Could you check a few things on this drawing? It's one solid part, dimensions in mm from its lowest x, y, z. A direction names the side the tool comes from. Give positions to 0.01 mm unless a question says otherwise; leave off trailing zeros. Order: outer loops, then holes, each group sorted by start corner. A loop starts at its lowest first (then second) coordinate and runs counter-clockwise, first axis right, second up.
Item 1: I want a section at D-D, the plane z = 12.5. Write out the boundary of the cut face in (x, y).
Item 2: I'm going to push flat-ended pins straight in: pin 1 Ø3.5 at (x, z) = (22, 7.5) entering from +Y; pin 2 Ø5 at (x, y) = (14.5, 12) entering from -Z. Where does each tip first touch, or does it pass through?
Item 3: I want a section at A-A, the plane y = 7.5. Write out the boundary of the cut face in (x, z), then the cut area to 3 significant figures.
Item 4: I want a section at B-B, the plane z = 2.4. Write out the boundary of the cut face in (x, y).
Item 5: Which directions (+Z, -Z, +X, -X, +Y, -Y) give clear straight access to the entire face, cutting with the end or side of a thin tool? Please do the marked faces 5, 6 and 7.
Item 6: I want a section at C-C, the plane x = 21. Write out the boundary of the cut face in (y, z), then the cut area to 3 significant figures.
Item 7: If I drill on line 1 along Z through (x, y) = (2.4, 1); line 2 along Z through (x, y) = (23.5, 15.5); line 3 along Y through (x, z) = (16.75, 13), over which ranges is the centre line in solid material (lowest first)?
Item 8: If we mould it in two halves opening along Z, with no side actions, what happens to the marked faces 1, 2, 3 and 4? For each: +Z half, -Z half, draft (parallel to the pull), parting line (faces both ways), or undercut.
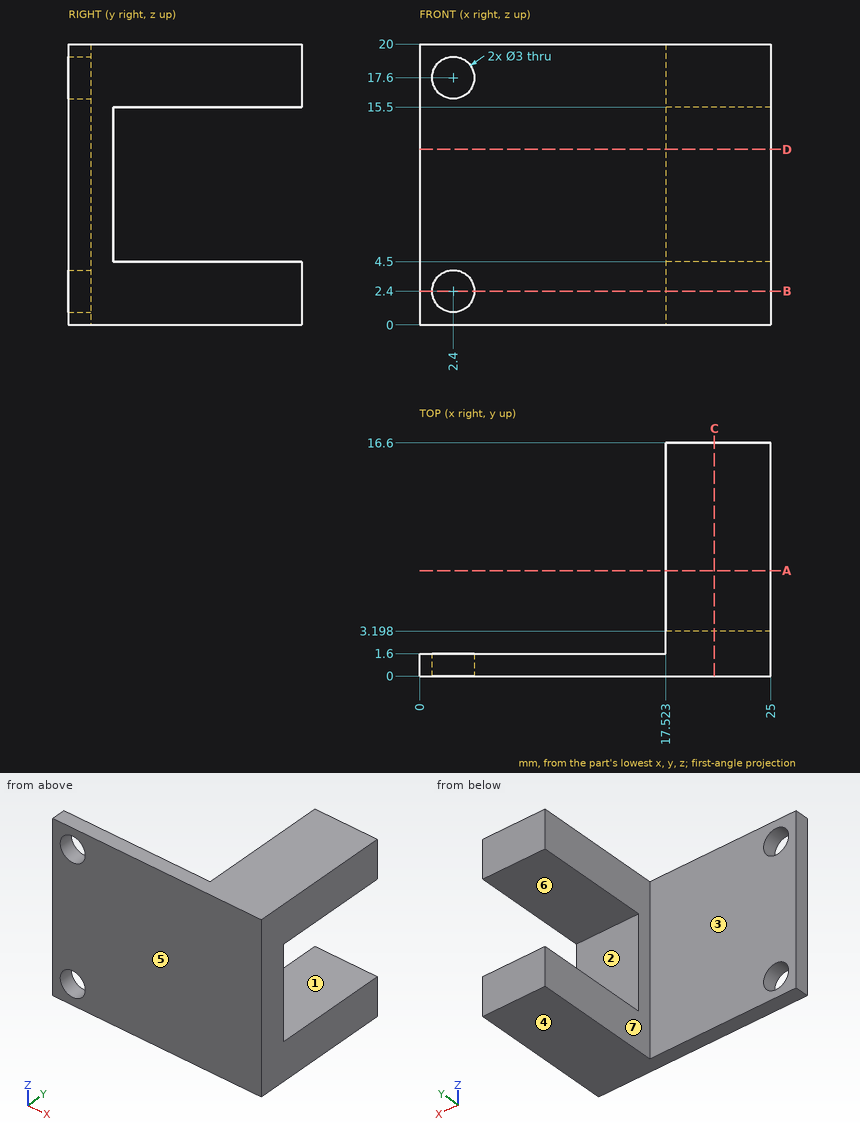
Results list:
1. outline: (0, 0) - (25, 0) - (25, 3.2) - (17.52, 3.2) - (17.52, 1.6) - (0, 1.6) - close
2. pin 1: stops at y = 3.2
2. pin 2: passes through
3. outline: (17.52, 0) - (25, 0) - (25, 4.5) - (17.52, 4.5) - close; (17.52, 15.5) - (25, 15.5) - (25, 20) - (17.52, 20) - close
3. area: 67.3 mm2
4. outline: (0, 0) - (0.9, 0) - (0.9, 1.6) - (0, 1.6) - close; (3.9, 0) - (25, 0) - (25, 16.6) - (17.52, 16.6) - (17.52, 1.6) - (3.9, 1.6) - close
5. face 5: +Z, -Z, +X, -X, -Y
5. face 6: +X, -X, +Y
5. face 7: +Z, -Z, -X, +Y
6. outline: (0, 0) - (16.6, 0) - (16.6, 4.5) - (3.2, 4.5) - (3.2, 15.5) - (16.6, 15.5) - (16.6, 20) - (0, 20) - close
6. area: 185 mm2
7. line 1: z = 0 to 0.9, 3.9 to 16.1, 19.1 to 20
7. line 2: z = 0 to 4.5, 15.5 to 20
7. line 3: y = 0 to 1.6
8. face 1: undercut
8. face 2: undercut
8. face 3: draft
8. face 4: -Z half
